For this review, use the dimensioned drawing (mm, ordinates from the lowest corner) and the shaded views. A direction names the side the tool comes from. Coordinates: 2 decimals unless noted, no trailing zeros. Loops run counter-clockwise (first coordinate to the right, second up) from the corner with the lowest first, then second, coordinate; pieces in that order, holes last. Notation, with made-up numbers: (47, -29.75) - (100, -29.75) arc R18 ccw to (100, -18.75) - close; hole circle Ø6 at (82, 35). An arc over 180 degrees is marked (long way). Answer in a Markdown table with one row per item. Add a question column.
(1) We need section A-A, the plane y = 12. Write out the cut boundary in (x, z).
(2) For the marked faces 4 and 5, list the 3-axis set-ups (+Z, -Z, +X, -X, +Y, -Y) from which the entire face can be reached by the end or side of a thin tool; tool diameter is ignored.
(3) We need section C-C, the plane x = 2. Write out the cut boundary in (y, z), plus the area to 3 significant figures.
(4) We need section D-D, the plane z = 19.75. Write out the cut boundary in (x, y), plus the area to 3 significant figures.
(5) To check wall thickness, follow L1, parallel to Z at x = 7.5, y = 12; L2, parallel to Z at x = 10.3, y = 12; L3, parallel to X at y = 16.5, z = 22.25. State the ranges of each line that lie inside material, in increasing order. Write a range as [from, to].
(6) The part is to be moulded in two halves that separate along Y. For the marked faces 1, 2 and 3, say which applies: released by +Y, released by -Y, zero draft, split by the parting line, or undercut.
(7) Clearance check with flat-ended pins moving along their axes: pin 1 (6 mm diameter, centred on x = 6, y = 8.5, fed in from -Z); pin 2 (6.5 mm diameter, centred on y = 12, z = 12, fed in from +X). State where each tip first meets the part, or that it passes through.
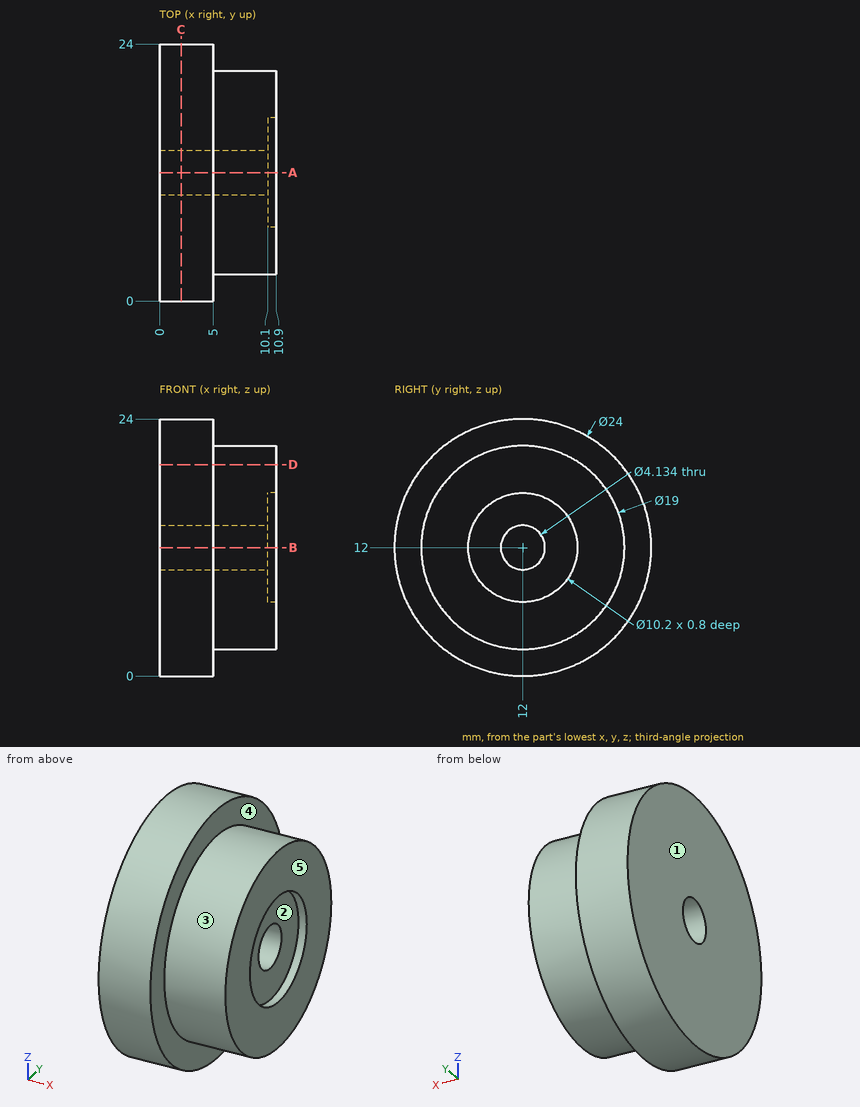
Responses:
| question | item | result |
|---|---|---|
| 1 | outline | (0, 0) - (5, 0) - (5, 2.5) - (10.9, 2.5) - (10.9, 6.9) - (10.1, 6.9) - (10.1, 9.93) - (0, 9.93) - close; (0, 14.07) - (10.1, 14.07) - (10.1, 17.1) - (10.9, 17.1) - (10.9, 21.5) - (5, 21.5) - (5, 24) - (0, 24) - close |
| 2 | face 4 | +X |
| 2 | face 5 | +Z, -Z, +X, +Y, -Y |
| 3 | outline | circle Ø24 at (12, 12); hole circle Ø4.13 at (12, 12) |
| 3 | area | 439 mm2 |
| 4 | outline | (0, 2.84) - (5, 2.84) - (5, 6.51) - (10.9, 6.51) - (10.9, 17.49) - (5, 17.49) - (5, 21.16) - (0, 21.16) - close |
| 4 | area | 156 mm2 |
| 5 | L1 | z = [2.5, 9.93], [14.07, 21.5] |
| 5 | L2 | z = [2.5, 6.9], [17.1, 21.5] |
| 5 | L3 | x = [0, 5] |
| 6 | face 1 | zero draft |
| 6 | face 2 | undercut |
| 6 | face 3 | split by the parting line |
| 7 | pin 1 | stops at z = 0.02 |
| 7 | pin 2 | stops at x = 10.1 |
